from build123d import *

# Parameters (mm, degrees)
SKETCH_1_R               = 10
EXTRUDE_351_DEPTH        = 2
SKETCH_2_R               = 4.5
EXTRUDE_436_DEPTH        = 2
SKETCH_3_R               = 3
CUT_EXTRUDE_526_DEPTH    = 3
SKETCH_4_R               = 1.5
CUT_EXTRUDE_623_DEPTH    = 15.456832295
SKETCH_5_R               = 1.5
CUT_EXTRUDE_727_DEPTH    = 15.282856857
PATTERN_CIRCULAR_1_COUNT = 4


with BuildPart() as part:
    # Эскиз1 → Extrude 351 (new body)
    with BuildSketch(Plane(origin=(0, 0, 0), x_dir=(1, 0, 0), z_dir=(0, 1, 0))):
        with Locations(Location((0, 0, 0), (0, 0, 270))):
            Circle(SKETCH_1_R)
    extrude(amount=EXTRUDE_351_DEPTH)

    # Эскиз2 → Extrude 436 (add)
    with BuildSketch(Plane(origin=(0, 2, 0), x_dir=(1, 0, 0), z_dir=(0, 1, 0))):
        with Locations(Location((0, 0, 0), (0, 0, 270))):
            Circle(SKETCH_2_R)
    extrude(amount=EXTRUDE_436_DEPTH)

    # Эскиз3 → Cut-Extrude 526 (cut)
    with BuildSketch(Plane(origin=(0, 4, 0), x_dir=(1, 0, 0), z_dir=(0, 1, 0))):
        with Locations(Location((0, 0, 0), (0, 0, 270))):
            Circle(SKETCH_3_R)
    extrude(amount=-CUT_EXTRUDE_526_DEPTH, mode=Mode.SUBTRACT)

    # Эскиз4 → Cut-Extrude 623 (cut, through all)
    with BuildSketch(Plane(origin=(0, 1, 0), x_dir=(1, 0, 0), z_dir=(0, 1, 0))):
        with Locations(Location((0, 0, 0), (0, 0, 270))):
            Circle(SKETCH_4_R)
    extrude(amount=-CUT_EXTRUDE_623_DEPTH, mode=Mode.SUBTRACT)

    # Эскиз5 → Cut-Extrude 727 (cut, through all)
    with BuildSketch(Plane(origin=(0, 2, 0), x_dir=(1, 0, 0), z_dir=(0, 1, 0))):
        with Locations(Location((7, 0, 0), (0, 0, 270))):
            Circle(SKETCH_5_R)
    cut_extrude_727 = extrude(amount=-CUT_EXTRUDE_727_DEPTH, mode=Mode.SUBTRACT)

    # Круговой массив1: Cut-Extrude 727 ×4 about axis
    pattern_circular_1_axis = Axis((0, 0, 0), (0, 1, 0))
    for i in range(1, PATTERN_CIRCULAR_1_COUNT):
        add(cut_extrude_727.rotate(pattern_circular_1_axis, i * 360 / PATTERN_CIRCULAR_1_COUNT), mode=Mode.SUBTRACT)


solid = part.part
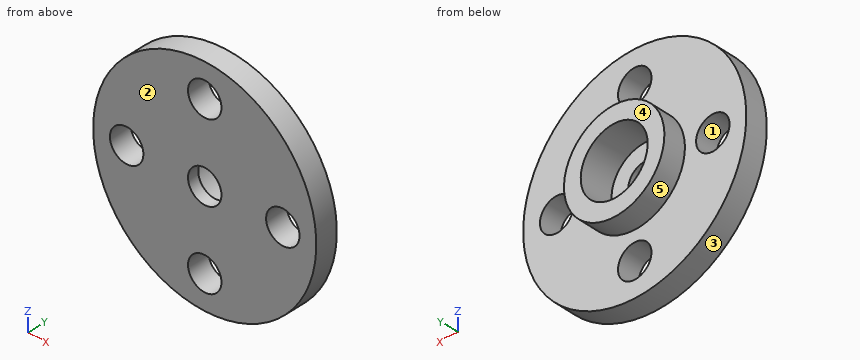
Work out the finished part from the listing and answer in its coordinate system (mm). Face numbers are marked on the shaded views. A direction names the side the tool comes from. Round coordinates to 2 decimals unless told otherwise and drop trailing zeros. Order: outer loops, then holes, each group sorted by start corner. A loop starts at its lowest first (then second) coordinate and runs counter-clockwise, first axis right, second up. Notation, with made-up numbers: M 12.25,10 L 60.25,10 A14 cw 60.25,28 Z; hole C 13.5,8.5 d3. An arc over 180 degrees is marked long. Put each result on its own line as item: value. Start each with the question number.
Q1. Section A-A, the plane x = 0 is taken. Write down the section's boundary in (y, z).
Q2. Section C-C, the plane z = -7.5 is taken. Write down the section's boundary in (x, y).
Q3. Section D-D, the plane x = 2.5 is taken. Write down the section's boundary in (y, z), and give its area (3 significant figures).
Q4. For a pull along X with two mould halves and no side action, classify the marked faces 1, 2 and 3 as pulls with the +X half, pulls with the -X half, needs draft (parallel to the pull), parting line crosses it, or undercut.
Q5. Straight lines are drawn through the part: L1, parallel to X at y = 0.5, z = 0; L2, parallel to X at y = 1.45, z = 0; L3, parallel to Y at x = -5.25, z = -7.75. For each, find the intervals that lie inside material, in ascending order. Write a range as [from, to].
Q6. Section B-B, the plane z = 1.25 is taken. Write down the section's boundary in (x, y), and give its area (3 significant figures).
Q7. Flat-ended cylindrical pins translate along their axes: pin 1 (9.5 mm diameter, centred on x = 0, z = 0, fed in from -Y); pin 2 (1.5 mm diameter, centred on x = -5.5, y = 1.5, fed in from +Z); pin 3 (4 mm diameter, centred on x = 0, z = 0, fed in from +Y). Find the tip coordinate at first contact, or state that the pin passes through.
Q8. A tool of negligible diameter and unlimited length cuts with its end or side. For the marked faces 4 and 5, from which of +Z, -Z, +X, -X, +Y, -Y can it reach the whole face along a straight path? Write none if from no direction.
Findings below:
1. outline: M 0,-10 L 2,-10 L 2,-8.5 L 0,-8.5 Z; M 0,-5.5 L 2,-5.5 L 2,-4.5 L 4,-4.5 L 4,-3 L 1,-3 L 1,-1.5 L 0,-1.5 Z; M 0,1.5 L 1,1.5 L 1,3 L 4,3 L 4,4.5 L 2,4.5 L 2,5.5 L 0,5.5 Z; M 0,8.5 L 2,8.5 L 2,10 L 0,10 Z
2. outline: M -6.61,0 L -1.41,0 L -1.41,2 L -6.61,2 Z; M 1.41,0 L 6.61,0 L 6.61,2 L 1.41,2 Z
3. outline: M 0,-9.68 L 2,-9.68 L 2,-3.74 L 4,-3.74 L 4,-1.66 L 1,-1.66 L 1,1.66 L 4,1.66 L 4,3.74 L 2,3.74 L 2,9.68 L 0,9.68 Z
3. area: 43.7 mm^2
4. face 1: undercut
4. face 2: needs draft
4. face 3: parting line crosses it
5. L1: x = [-10, -8.5], [-5.5, -1.5], [1.5, 5.5], [8.5, 10]
5. L2: x = [-10, -8.5], [-5.5, -3], [3, 5.5], [8.5, 10]
5. L3: y = [0, 2]
6. outline: M -9.92,0 L -7.83,0 L -7.83,2 L -9.92,2 Z; M -6.17,0 L -0.83,0 L -0.83,1 L -2.73,1 L -2.73,4 L -4.32,4 L -4.32,2 L -6.17,2 Z; M 0.83,0 L 6.17,0 L 6.17,2 L 4.32,2 L 4.32,4 L 2.73,4 L 2.73,1 L 0.83,1 Z; M 7.83,0 L 9.92,0 L 9.92,2 L 7.83,2 Z
6. area: 32.3 mm^2
7. pin 1: stops at y = 0
7. pin 2: stops at z = 8.8
7. pin 3: stops at y = 1
8. face 4: +Z, -Z, +X, -X, +Y
8. face 5: +Y
